from build123d import *

# Parameters (mm, degrees)
SKETCH1_W           = 203.2
SKETCH1_H           = 152.4
BOSS_EXTRUDE1_DEPTH = 3.175
SKETCH5_R           = 9.5504
SKETCH5_R_2         = 2.54
CUT_EXTRUDE4_DEPTH  = 4.7625
SKETCH6_R           = 14.29004
CUT_EXTRUDE5_DEPTH  = 4.7625
SKETCH4_R           = 3.175
CUT_EXTRUDE7_DEPTH  = 5.08
SKETCH7_R           = 14.2875
CUT_EXTRUDE8_DEPTH  = 25.4


with BuildPart() as part:
    # Sketch1 → Boss-Extrude1 (new body)
    with BuildSketch(Plane(origin=(0, 0, 0), x_dir=(1, 0, 0), z_dir=(0, 1, 0))):
        with Locations((101.6, 76.2)):
            Rectangle(SKETCH1_W, SKETCH1_H)
    extrude(amount=BOSS_EXTRUDE1_DEPTH)

    # Sketch5 → Cut-Extrude4 (cut)
    with BuildSketch(Plane(origin=(0, 3.175, 0), x_dir=(1, 0, 0), z_dir=(0, 1, 0))):
        with Locations(Location((50.8, 54.1274, 0), (0, 0, 270))):  # turned: the seam where the file's is
            Circle(SKETCH5_R)
        with Locations(Location((32.8422, 72.0852, 0), (0, 0, 270))):  # turned: the seam where the file's is
            Circle(SKETCH5_R_2)
        with Locations(Location((68.7578, 36.1696, 0), (0, 0, 270))):  # turned: the seam where the file's is
            Circle(SKETCH5_R_2)
    extrude(amount=-CUT_EXTRUDE4_DEPTH, mode=Mode.SUBTRACT)

    # Sketch6 → Cut-Extrude5 (cut)
    with BuildSketch(Plane(origin=(0, 3.175, 0), x_dir=(1, 0, 0), z_dir=(0, 1, 0))):
        with Locations(Location((82.55, 82.55, 0), (0, 0, 270))):  # turned: the seam where the file's is
            Circle(SKETCH6_R)
    extrude(amount=-CUT_EXTRUDE5_DEPTH, mode=Mode.SUBTRACT)

    # Sketch4 → Cut-Extrude7 (cut)
    with BuildSketch(Plane(origin=(0, 3.175, 0), x_dir=(1, 0, 0), z_dir=(0, 1, 0))):
        with Locations(Location((12.7, 12.7, 0), (0, 0, 270))):  # turned: the seam where the file's is
            Circle(SKETCH4_R)
        with Locations(Location((38.1, 12.7, 0), (0, 0, 270))):  # turned: the seam where the file's is
            Circle(SKETCH4_R)
        with Locations(Location((63.5, 12.7, 0), (0, 0, 270))):  # turned: the seam where the file's is
            Circle(SKETCH4_R)
        with Locations(Location((88.9, 12.7, 0), (0, 0, 270))):  # turned: the seam where the file's is
            Circle(SKETCH4_R)
        with Locations(Location((114.3, 12.7, 0), (0, 0, 270))):  # turned: the seam where the file's is
            Circle(SKETCH4_R)
        with Locations(Location((139.7, 12.7, 0), (0, 0, 270))):  # turned: the seam where the file's is
            Circle(SKETCH4_R)
        with Locations(Location((165.1, 12.7, 0), (0, 0, 270))):  # turned: the seam where the file's is
            Circle(SKETCH4_R)
        with Locations(Location((190.5, 12.7, 0), (0, 0, 270))):  # turned: the seam where the file's is
            Circle(SKETCH4_R)
        with Locations(Location((12.7, 38.1, 0), (0, 0, 270))):  # turned: the seam where the file's is
            Circle(SKETCH4_R)
        with Locations(Location((12.7, 63.5, 0), (0, 0, 270))):  # turned: the seam where the file's is
            Circle(SKETCH4_R)
        with Locations(Location((12.7, 88.9, 0), (0, 0, 270))):  # turned: the seam where the file's is
            Circle(SKETCH4_R)
        with Locations(Location((12.7, 114.3, 0), (0, 0, 270))):  # turned: the seam where the file's is
            Circle(SKETCH4_R)
        with Locations(Location((12.7, 139.7, 0), (0, 0, 270))):  # turned: the seam where the file's is
            Circle(SKETCH4_R)
        with Locations(Location((38.1, 139.7, 0), (0, 0, 270))):  # turned: the seam where the file's is
            Circle(SKETCH4_R)
        with Locations(Location((63.5, 139.7, 0), (0, 0, 270))):  # turned: the seam where the file's is
            Circle(SKETCH4_R)
        with Locations(Location((88.9, 139.7, 0), (0, 0, 270))):  # turned: the seam where the file's is
            Circle(SKETCH4_R)
        with Locations(Location((114.3, 139.7, 0), (0, 0, 270))):  # turned: the seam where the file's is
            Circle(SKETCH4_R)
        with Locations(Location((190.5, 114.3, 0), (0, 0, 270))):  # turned: the seam where the file's is
            Circle(SKETCH4_R)
        with Locations(Location((190.5, 139.7, 0), (0, 0, 270))):  # turned: the seam where the file's is
            Circle(SKETCH4_R)
    extrude(amount=-CUT_EXTRUDE7_DEPTH, mode=Mode.SUBTRACT)

    # Sketch7 → Cut-Extrude8 (cut)
    with BuildSketch(Plane(origin=(0, 3.175, 0), x_dir=(1, 0, 0), z_dir=(0, 1, 0))):
        with Locations(Location((125.095, 110.49, 0), (0, 0, 270))):  # turned: the seam where the file's is
            Circle(SKETCH7_R)
        with Locations(Location((131.7498, 53.34, 0), (0, 0, 270))):  # turned: the seam where the file's is
            Circle(SKETCH7_R)
    extrude(amount=-CUT_EXTRUDE8_DEPTH, mode=Mode.SUBTRACT)


solid = part.part
Verification items for the finished model (mm, model axes). Round coordinates to 2 decimals unless told otherwise and drop trailing zeros. Write each loop counter-clockwise with the first axis right and the second up, starting at its lowest first coordinate (ties: lowest second). Pieces come first, ordered by that corner, then holes.
(1) Depth check by flat-ended pin: pin 1 Ø7.5 at (x, z) = (165.1, -12.7) entering from -Y. Enter the tip coordinate at first touch or a pass-through.
Returned:
pin 1: stops at y = 0
(2) Material ranges on line 1 (X direction, y = 2.25, z = -53); line 2 (Z direction, x = 115, y = 2.1); line 3 (Z direction, x = 126, y = 1.25), recorded low to high.
Returned:
line 1: x = 0 to 41.32, 60.28 to 117.47, 146.03 to 203.2
line 2: z = -152.4 to -142.8, -136.6 to -120.6, -100.38 to -15.8, -9.6 to 0
line 3: z = -152.4 to -124.75, -96.23 to -66.42, -40.26 to 0
(3) Section check B-B (z = -88.9). Enter the section's corners in (x, y) (3 decimals), plus the area to 3 significant figures.
Returned:
outline: (0, 0) - (9.525, 0) - (9.525, 3.175) - (0, 3.175) - close; (15.875, 0) - (69.748, 0) - (69.748, 3.175) - (15.875, 3.175) - close; (95.352, 0) - (203.2, 0) - (203.2, 3.175) - (95.352, 3.175) - close
area: 544 mm2
(4) Section check C-C (z = -114.3). Enter the section's corners in (x, y) (3 decimals).
Returned:
outline: (0, 0) - (9.525, 0) - (9.525, 3.175) - (0, 3.175) - close; (15.875, 0) - (111.325, 0) - (111.325, 3.175) - (15.875, 3.175) - close; (138.865, 0) - (187.325, 0) - (187.325, 3.175) - (138.865, 3.175) - close; (193.675, 0) - (203.2, 0) - (203.2, 3.175) - (193.675, 3.175) - close
(5) Section check A-A (x = 50.8). Enter the section's corners in (y, z) (3 decimals).
Returned:
outline: (0, -152.4) - (3.175, -152.4) - (3.175, -63.678) - (0, -63.678) - close; (0, -44.577) - (3.175, -44.577) - (3.175, 0) - (0, 0) - close
(6) Section check D-D (y = 0.75). Give the number of separate pieces and of enclosed holes in the cut face, plus the area to 3 significant figures.
Returned:
separate pieces: 1
enclosed holes: 25
area: 28,100 mm2
(7) Mould release check, pull along X, two halves, no side actions. Record for faces 1 (the flat face through (100, 3.175, -77)), 2 (the cylindrical face through (142.85, 1.61, -13.11)): pulls with the +X half, pulls with the -X half, needs draft (parallel to the pull), parting line crosses it, or undercut.
Returned:
face 1: needs draft
face 2: undercut
